Autodesk Inventor part; units mm, degrees
ref_plane "YZ Plane" through (0, 0, 0) normal (1, 0, 0) x (0, 1, 0)
ref_plane "XZ Plane" through (0, 0, 0) normal (0, 1, 0) x (-1, 0, 0)
ref_plane "XY Plane" through (0, 0, 0) normal (0, 0, 1) x (1, 0, 0)
sketch "Sketch1" plane through (0, 0, 0) normal (0, 0, 1) x (1, 0, 0)
  circle A0 centre (4, 4) radius 1.2
  circle A1 centre (4, 4) radius 2
  point P0 (0, 0)
  dimension "d0" = 4
extrude "Extrusion1" add sketch "Sketch1" against normal blind 12 contours A0 | A1
sketch "Sketch2" plane through (4, 4, 0) normal (0, 0, 1) x (1, 0, 0)
  circle A0 centre (0, 0) radius 2
  circle A1 centre (0, 0) radius 3.65
  point P0 (-4, -4)
  dimension "d3" = 7.3
extrude "Extrusion2" add sketch "Sketch2" along normal blind 2.3 contours A0 | A1
fillet "Fillet1" radius 2.2 1 edges at (0.35, 4, 2.3)
sketch "Sketch4" plane through (4, 4, 2.3) normal (0, 0, 1) x (1, 0, 0)
  circle A0 centre (0, 0) radius 1.45
  line L0 (0.7217, 1.25) -> (1.4434, 0)
  line L1 (1.4434, 0) -> (0.7217, -1.25)
  line L2 (0.7217, -1.25) -> (-0.7217, -1.25)
  line L3 (-0.7217, -1.25) -> (-1.4434, 0)
  line L4 (-1.4434, 0) -> (-0.7217, 1.25)
  line L5 (-0.7217, 1.25) -> (0.7217, 1.25)
  point P0 (-4, -4)
  dimension "d10" = 2.5
extrude "Extrusion4" cut sketch "Sketch4" along normal mid plane 4 contours L0 L1 L2 L3 L4 L5
thread "Thread1"
properties part number "m3 6" material "Steel"
The model under review builds one solid part; all positions refer to its coordinate system, in mm. A direction names the side the tool comes from. Round coordinates to 2 decimals unless told otherwise and drop trailing zeros. Loops run counter-clockwise (first coordinate to the right, second up) from the corner with the lowest first, then second, coordinate; pieces in that order, holes last. Notation, with made-up numbers: M 42,69 L 74,69 A28 cw 74,96 Z; hole C 24.5,-20 d7. An arc over 180 degrees is marked long. Put each result on its own line as item: value.
Q1. To check wall thickness, follow L1, parallel to Y at x = 4, z = -7.75; L2, parallel to X at y = 2, z = 1.25; L3, parallel to Z at x = 6.25, y = 4.75. State the ranges of each line that lie inside material, in increasing order.
Result set:
L1: y = 2 to 6
L2: x = 1.34 to 6.66
L3: z = 0 to 2.1
Q2. Consider section A-A, the plane z = -5.75. Give the boundary of the cut face in (x, y), then the cut area to 3 significant figures.
Result set:
outline: C 4,4 d4
area: 12.6 mm²
Q3. Machinability: for faces 5 (the flat face through (5.088, 3.384, 1.286)), 6 (the flat face through (4, 4, -12)), which of the approach directions +Z, -Z, +X, -X, +Y, -Y give a long, thin tool a straight path to every point of the face, cutting with its end or side? Answer none if there is none.
Result set:
face 5: +Z
face 6: -Z, +X, -X, +Y, -Y
Q4. Mouldability with a two-part tool opening along X and no side actions: class faces 1 (the cylindrical face through (2.4, 2.8, -5.9)), 2 (the flat face through (4, 2.75, 1)), 3 (the flat face through (6, 2, 0)), 4 (the flat face through (2.92, 3.37, 1.29)) as released by +X, released by -X, zero draft, split by the parting line, or undercut.
Result set:
face 1: split by the parting line
face 2: undercut
face 3: zero draft
face 4: undercut
Q5. For pin 1 (2 mm diameter, centred on x = 4.5, y = 4.5, fed in from +Z); pin 2 (1.5 mm diameter, centred on x = 4, z = -8.5, fed in from -Y); pin 3 (2 mm diameter, centred on x = 2, y = 1, fed in from -Z); pin 4 (0.7 mm diameter, centred on x = 4, z = 1.5, fed in from -Y), all flat-tipped, find the tip position at first contact; note any pin that passes through.
Result set:
pin 1: stops at z = 2.3
pin 2: stops at y = 2
pin 3: stops at z = 0
pin 4: stops at y = 0.62
